Check sheet for the modelled part. Datum: model origin and axes. Units: mm. A direction names the side the tool comes from. Round coordinates to 2 decimals unless told otherwise and drop trailing zeros. Write each loop counter-clockwise with the first axis right and the second up, starting at its lowest first coordinate (ties: lowest second). Pieces come first, ordered by that corner, then holes. Notation, with made-up numbers: M 51.5,55 L 87.5,55 A17 cw 87.5,69 Z; hole C -28,58 d3. An arc over 180 degrees is marked long. Answer in a Markdown table with one row per item.
```python
from build123d import *

# Parameters (mm, degrees)
F0_W      = 90.29606
F0_H      = 26.348686
F1_DEPTH  = 50
F2_W      = 29.309216
F2_H      = 88.519738
F3_DEPTH  = 25
F4_R      = 8.4699
F5_DEPTH  = 25
F6_R      = 5.178495
F7_DEPTH  = 70
F8_R      = 5.283524
F9_DEPTH  = 40
F12_R     = 11.126617
F13_DEPTH = 6


with BuildPart() as f1:
    # F0 (on Front) → F1 (new body)
    with BuildSketch(Plane.XZ):
        Rectangle(F0_W, F0_H)
    extrude(amount=F1_DEPTH)

    # F2 (on Front) → F3 (join)
    with BuildSketch(Plane.XZ):
        Rectangle(F2_W, F2_H)
    extrude(amount=-F3_DEPTH)



with BuildPart() as f5:
    # F4 (on Front) → F5 (new body)
    with BuildSketch(Plane.XZ):
        Circle(F4_R)
    extrude(amount=F5_DEPTH)


with BuildPart() as f1_1:
    add(f1.part)

    add(f5.part)  # F7 merges F5
    # F6 (on Front) → F7 (join)
    with BuildSketch(Plane.XZ):
        Circle(F6_R)
    extrude(amount=F7_DEPTH)

    # F8 (on Front) → F9 (join)
    with BuildSketch(Plane.XZ):
        Circle(F8_R)
    extrude(amount=-F9_DEPTH)

    # F12 (on offset) → F13 (join)
    with BuildSketch(Plane.XZ.offset(75)):
        Circle(F12_R)
    extrude(amount=-F13_DEPTH)


solid = f1_1.part
```
1. Section check A-A, the plane z = -9. Record the cut outline in (x, y).
Found:
| item | result |
|---|---|
| outline | M -45.15,-50 L 45.15,-50 L 45.15,0 L 14.65,0 L 14.65,25 L -14.65,25 L -14.65,0 L -45.15,0 Z; M -6.54,-75 L 6.54,-75 L 6.54,-69 L -6.54,-69 Z |
2. Go/stop test with flat-tipped pins: pin 1 (6 mm diameter, centred on x = 8, z = -17.5, fed in from -Y); pin 2 (3 mm diameter, centred on x = -4, z = -7, fed in from +Y); pin 3 (25 mm diameter, centred on x = -6, y = -14, fed in from -Z). Record where each tip stops, or that it passes through.
Found:
| item | result |
|---|---|
| pin 1 | stops at y = 0 |
| pin 2 | stops at y = 25 |
| pin 3 | stops at z = -13.17 |
3. Section check C-C, the plane z = 0. Record the cut outline in (x, y), and give its area (3 significant figures).
Found:
| item | result |
|---|---|
| outline | M -45.15,-50 L -5.18,-50 L -5.18,-69 L -11.13,-69 L -11.13,-75 L 11.13,-75 L 11.13,-69 L 5.18,-69 L 5.18,-50 L 45.15,-50 L 45.15,0 L 14.65,0 L 14.65,25 L 5.28,25 L 5.28,40 L -5.28,40 L -5.28,25 L -14.65,25 L -14.65,0 L -45.15,0 Z |
| area | 5,740 mm2 |
4. Access from +Z, -Z, +X, -X, +Y, -Y to the whole of each face (thin tool, end or side, straight path). Record for faces 5 (the face through (-30, 0, 0)), 6 (the face through (-1, -25, 13.174)), 7 (the face through (14.655, 12, -1)), 8 (the face through (10.613, -72.042, 3.342)), 9 (the face through (5.04, 32.39, 1.59)).
Found:
| item | result |
|---|---|
| face 5 | +Z, -Z, -X, +Y |
| face 6 | +Z, +X, -X, -Y |
| face 7 | +Z, -Z, +X, +Y |
| face 8 | -Y |
| face 9 | +Y |
5. Section check D-D, the plane y = 11.5. Record the cut outline in (x, z), and give its area (3 significant figures).
Found:
| item | result |
|---|---|
| outline | M -14.65,-44.26 L 14.65,-44.26 L 14.65,44.26 L -14.65,44.26 Z |
| area | 2,590 mm2 |
6. Section check B-B, the plane x = -7.5. Record the cut outline in (y, z), and give its area (3 significant figures).
Found:
| item | result |
|---|---|
| outline | M -75,-8.22 L -69,-8.22 L -69,8.22 L -75,8.22 Z; M -50,-13.17 L 0,-13.17 L 0,-44.26 L 25,-44.26 L 25,44.26 L 0,44.26 L 0,13.17 L -50,13.17 Z |
| area | 3,630 mm2 |
7. Scan lines: L1, parallel to Y at x = 4.5, z = -6.5; L2, parallel to X at y = 4, z = 5; L3, parallel to Z at x = -7, y = -29.5. Record each from-to range of solid material in increasing order.
Found:
| item | result |
|---|---|
| L1 | y = -75 to -69, -50 to 25 |
| L2 | x = -14.65 to 14.65 |
| L3 | z = -13.17 to 13.17 |
8. Draft check along Y on faces 1 (the face through (5, -69, -2)), 2 (the face through (0, 40, 0)), 3 (the face through (4.94, -59.37, 1.56)), 4 (the face through (0, 12, 44.26)). Enter one of: +Y half, -Y half, draft (parallel to the pull), parting line (faces both ways), or undercut.
Found:
| item | result |
|---|---|
| face 1 | undercut |
| face 2 | +Y half |
| face 3 | undercut |
| face 4 | draft |
